from build123d import *

# Parameters (mm, degrees)
SKETCH1_W           = 91
SKETCH1_H           = 61
BOSS_EXTRUDE1_DEPTH = 35
SKETCH2_R           = 1.25
CUT_EXTRUDE1_DEPTH  = 8
CUT_EXTRUDE2_START  = -83
SKETCH2_2_R         = 1.25
CUT_EXTRUDE2_DEPTH  = 8
FILLET2_R           = 3
CHAMFER1_SIZE       = 3
SKETCH3_R           = 1.25
CUT_EXTRUDE3_DEPTH  = 10


with BuildPart() as part:
    # Sketch1 → Boss-Extrude1 (new body)
    with BuildSketch(Plane(origin=(0, 0, 0), x_dir=(1, 0, 0), z_dir=(0, 1, 0))):
        with Locations((-45.5, -30.5)):
            Rectangle(SKETCH1_W, SKETCH1_H)
    extrude(amount=BOSS_EXTRUDE1_DEPTH)

    # Sketch2 → Cut-Extrude1 (cut)
    with BuildSketch(Plane(origin=(0, 0, 0), x_dir=(0, 0, -1), z_dir=(1, 0, 0))):
        with Locations((-8, 28)):
            Circle(SKETCH2_R)
        with Locations((-8, 3)):
            Circle(SKETCH2_R)
        with Locations(Location((-53, 3, 0), (0, 0, 180))):
            Circle(SKETCH2_R)
        with Locations(Location((-53, 28, 0), (0, 0, 180))):
            Circle(SKETCH2_R)
    extrude(amount=-CUT_EXTRUDE1_DEPTH, mode=Mode.SUBTRACT)

    # Sketch2<2> → Cut-Extrude2 (cut)
    with BuildSketch(Plane(origin=(0, 0, 0), x_dir=(0, 0, -1), z_dir=(1, 0, 0)).offset(CUT_EXTRUDE2_START)):
        with Locations((-8, 28)):
            Circle(SKETCH2_2_R)
        with Locations((-8, 3)):
            Circle(SKETCH2_2_R)
        with Locations(Location((-53, 3, 0), (0, 0, 180))):
            Circle(SKETCH2_2_R)
        with Locations(Location((-53, 28, 0), (0, 0, 180))):
            Circle(SKETCH2_2_R)
    extrude(amount=-CUT_EXTRUDE2_DEPTH, mode=Mode.SUBTRACT)

    # Fillet2
    fillet2_edges = [part.edges().sort_by_distance(p)[0] for p in [
        (0, 17.5, 61),
        (-91, 17.5, 61),
        (-91, 17.5, 0),
        (0, 17.5, 0),
    ]]
    fillet(fillet2_edges, radius=FILLET2_R)

    # Chamfer1
    chamfer1_edges = [part.edges().sort_by_distance(p)[0] for p in [
        (-91, 35, 30.5),
        (-45.5, 35, 0),
        (0, 35, 30.5),
        (-45.5, 35, 61),
        (-90.121320344, 35, 60.121320344),
        (-0.878679656, 35, 60.121320344),
        (-0.878679656, 35, 0.878679656),
        (-90.121320344, 35, 0.878679656),
    ]]
    chamfer(chamfer1_edges, length=CHAMFER1_SIZE)

    # Sketch3 → Cut-Extrude3 (cut)
    with BuildSketch(Plane.XZ):
        with Locations(Location((-45.5, 44.5, 0), (0, 0, 270))):
            Circle(SKETCH3_R)
        with Locations(Location((-45.5, 16.5, 0), (0, 0, 270))):
            Circle(SKETCH3_R)
    extrude(amount=-CUT_EXTRUDE3_DEPTH, mode=Mode.SUBTRACT)


solid = part.part
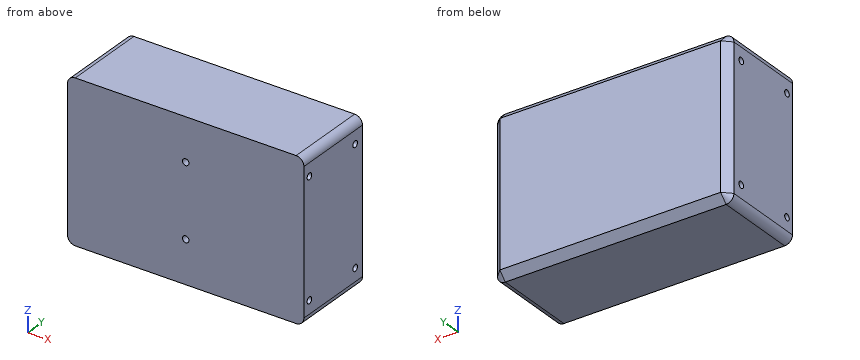
Source: CAD feature listing. Evaluate the final solid. Frame: model axes, mm. Coordinates: 2 decimals unless noted, no trailing zeros. Order: outer loops, then holes, each group sorted by start corner. A loop starts at its lowest first (then second) coordinate and runs counter-clockwise, first axis right, second up. Notation, with made-up numbers: M -32.75,69.25 L -3.75,69.25 A35 cw -3.75,103.25 Z; hole C 17,32 d2. An arc over 180 degrees is marked long. Write each question's results on one line, items separated by ' | '. Start each with the question number.
1. Section A-A, the plane y = 3. Return the cut outline in (x, z), then the cut area to 3 significant figures.
2. Material intervals for L1, parallel to Y at x = -88, z = 8; L2, parallel to X at y = 4, z = 44.5; L3, parallel to Z at x = -45, y = 7, sorted ascending.
3. Section B-B, the plane x = -45.5. Return the cut outline in (y, z).
4. Section C-C, the plane z = 53. Return the cut outline in (x, y).
5. Pin query (flat end, axial travel): pin 1 (2 mm diameter, centred on y = 3, z = 53, fed in from -X); pin 2 (2 mm diameter, centred on y = 3, z = 53, fed in from +X); pin 3 (1.2 mm diameter, centred on x = -46, z = 44.5, fed in from -Y). Return the tip coordinate at first contact, or that it passes through.
Solution:
1) outline: M -91,3 A3 ccw -88,0 L -3,0 A3 ccw 0,3 L 0,6.75 L -8,6.75 L -8,9.25 L 0,9.25 L 0,51.75 L -8,51.75 L -8,54.25 L 0,54.25 L 0,58 A3 ccw -3,61 L -88,61 A3 ccw -91,58 L -91,54.25 L -83,54.25 L -83,51.75 L -91,51.75 L -91,9.25 L -83,9.25 L -83,6.75 L -91,6.75 Z; hole C -45.5,16.5 d2.5; hole C -45.5,44.5 d2.5 | area: 5,450 mm²
2) L1: 0 to 1.75, 4.25 to 26.75, 29.25 to 35 | L2: -91 to -46.75, -44.25 to 0 | L3: 0 to 15.35, 17.65 to 43.35, 45.65 to 61
3) outline: M 0,0 L 32,0 L 35,3 L 35,58 L 32,61 L 0,61 L 0,45.75 L 10,45.75 L 10,43.25 L 0,43.25 L 0,17.75 L 10,17.75 L 10,15.25 L 0,15.25 Z
4) outline: M -91,0 L 0,0 L 0,1.75 L -8,1.75 L -8,4.25 L 0,4.25 L 0,26.75 L -8,26.75 L -8,29.25 L 0,29.25 L 0,32 L -3,35 L -88,35 L -91,32 L -91,29.25 L -83,29.25 L -83,26.75 L -91,26.75 L -91,4.25 L -83,4.25 L -83,1.75 L -91,1.75 Z
5) pin 1: x = -83 | pin 2: x = -8 | pin 3: y = 10
